Check sheet for the modelled part. Datum: model origin and axes. Units: mm. A direction names the side the tool comes from. Give positions to 0.01 mm unless a question says otherwise; leave off trailing zeros. Loops run counter-clockwise (first coordinate to the right, second up) from the corner with the lowest first, then second, coordinate; pieces in that order, holes last. Notation, with made-up numbers: M 66.25,43.25 L 116.25,43.25 A16 cw 116.25,51.25 Z; hole C -12.75,78.25 d10. An arc over 180 degrees is marked long. Write each question's results on one line, items separated by ' | '. Start each with the question number.
1. Sectioned sample at A-A on y = 38.5. Record the cut outline in (x, z), and give its area (3 significant figures).
2. Tool access check on faces 4 (the flat face through (46, 3, -12.35)), 5 (the flat face through (7, 56, -9)), 6 (the flat face through (-1, 7, -7.5)), 7 (the flat face through (-35, 82, 25)). Record the directions out of +Z, -Z, +X, -X, +Y, -Y that give a thin tool (end or side, any length) a straight path to the whole face; none if there is none.
3. Sectioned sample at B-B on y = 76.5. Record the cut outline in (x, z), and give its area (3 significant figures).
4. Draft check along X on faces 1 (the cylindrical face through (6.3, 56.74, -8.23)), 2 (the flat face through (-30, 87, 30)), 3 (the flat face through (35, 82, -25)). Enter one of: pulls with the +X half, pulls with the -X half, needs draft (parallel to the pull), parting line crosses it, or undercut.
5. Material ranges on line 1 along X through (y, z) = (29, 1); line 2 along X through (y, z) = (60, -33); line 3 along Y through (x, z) = (-31.5, 10), recorded low to high.
6. Go/stop test with flat-tipped pins: pin 1 (3 mm diameter, centred on x = -19.5, z = -3, fed in from -Y); pin 2 (6 mm diameter, centred on x = 12, z = -2, fed in from +Y); pin 3 (3.5 mm diameter, centred on x = 45.5, y = 2.5, fed in from -Z). Record where each tip stops, or that it passes through.
7. Sectioned sample at C-C on y = 13.5. Record the cut outline in (x, z).
8. Sectioned sample at D-D on z = -2. Record the cut outline in (x, y).
```python
from build123d import *

# Parameters (mm, degrees)
SKETCH1_W            = 100
SKETCH1_H            = 100
BOSS_EXTRUDE1_DEPTH  = 25
SKETCH2_W            = 100
SKETCH2_H            = 100
SKETCH2_W_2          = 80
SKETCH2_H_2          = 80
BOSS_EXTRUDE2_DEPTH  = 40
SKETCH3_R            = 5
SKETCH3_W            = 15
SKETCH3_H            = 12
CUT_EXTRUDE1_DEPTH   = 130.325171564
FILLET2_R            = 10
FILLET3_R            = 10
FILLET4_R            = 10
FILLET5_R            = 10
BOSS_EXTRUDE3_DEPTH  = 15
SKETCH6_R            = 35
CUT_EXTRUDE3_DEPTH   = 25
SKETCH7_R            = 40.1
CUT_EXTRUDE4_DEPTH   = 10
BOSS_EXTRUDE4_DEPTH  = 12
SKETCH10_R           = 1.1
SKETCH10_W           = 5
SKETCH10_H           = 13.6
CUT_EXTRUDE5_DEPTH   = 10
FILLET6_R            = 5
SKETCH11_W           = 12
SKETCH11_H           = 0.5
CUT_EXTRUDE6_DEPTH   = 24
SKETCH12_W           = 10
SKETCH12_H           = 15
CUT_EXTRUDE7_DEPTH   = 24
SKETCH15_W           = 10
SKETCH15_H           = 2.75
BOSS_EXTRUDE5_DEPTH  = 5.4
SKETCH18_R           = 2.5
CUT_EXTRUDE8_DEPTH   = 7
BOSS_EXTRUDE6_DEPTH  = 5
FILLET8_R            = 3
FILLET8_OF_MIRROR3_R = 3


with BuildPart() as part:
    # Sketch1 → Boss-Extrude1 (new body)
    with BuildSketch(Plane(origin=(0, 0, 0), x_dir=(1, 0, 0), z_dir=(0, 1, 0))):
        Rectangle(SKETCH1_W, SKETCH1_H)
    extrude(amount=BOSS_EXTRUDE1_DEPTH)

    # Sketch2 → Boss-Extrude2 (add)
    with BuildSketch(Plane(origin=(0, 25, 0), x_dir=(1, 0, 0), z_dir=(0, 1, 0))):
        Rectangle(SKETCH2_W, SKETCH2_H)
        Rectangle(SKETCH2_W_2, SKETCH2_H_2, mode=Mode.SUBTRACT)
    extrude(amount=BOSS_EXTRUDE2_DEPTH)

    # Sketch3 → Cut-Extrude1 (cut, through all)
    with BuildSketch(Plane.ZY.offset(50)):
        with Locations((-25, 12)):
            Circle(SKETCH3_R)
        with Locations((25.313920598, 12)):
            Circle(SKETCH3_R)
        with Locations((0, 6)):
            Rectangle(SKETCH3_W, SKETCH3_H)
    extrude(amount=-CUT_EXTRUDE1_DEPTH, mode=Mode.SUBTRACT)

    # Fillet2
    fillet2_edges = [part.edges().sort_by_distance(p)[0] for p in [
        (50, 32.5, 50),
    ]]
    fillet(fillet2_edges, radius=FILLET2_R)

    # Fillet3
    fillet3_edges = [part.edges().sort_by_distance(p)[0] for p in [
        (50, 32.5, -50),
    ]]
    fillet(fillet3_edges, radius=FILLET3_R)

    # Fillet4
    fillet4_edges = [part.edges().sort_by_distance(p)[0] for p in [
        (-50, 32.5, -50),
    ]]
    fillet(fillet4_edges, radius=FILLET4_R)

    # Fillet5
    fillet5_edges = [part.edges().sort_by_distance(p)[0] for p in [
        (-50, 32.5, 50),
    ]]
    fillet(fillet5_edges, radius=FILLET5_R)

    # Sketch5 → Boss-Extrude3 (add)
    with BuildSketch(Plane(origin=(0, 65, 0), x_dir=(1, 0, 0), z_dir=(0, 1, 0))):
        with BuildLine():
            Line((-50, 40), (-50, -40))
            ThreePointArc((-50, -40), (-47.071067812, -47.071067812), (-40, -50))
            Line((-40, -50), (40, -50))
            ThreePointArc((40, -50), (47.071067812, -47.071067812), (50, -40))
            Line((50, -40), (50, 40))
            ThreePointArc((50, 40), (47.071067812, 47.071067812), (40, 50))
            Line((40, 50), (-40, 50))
            ThreePointArc((-40, 50), (-47.071067812, 47.071067812), (-50, 40))
        make_face()
    extrude(amount=BOSS_EXTRUDE3_DEPTH)

    # Sketch6 → Cut-Extrude3 (cut)
    with BuildSketch(Plane(origin=(0, 80, 0), x_dir=(1, 0, 0), z_dir=(0, 1, 0))):
        with Locations(Location((0.142992369, 0, 0), (0, 0, 270))):
            Circle(SKETCH6_R)
    extrude(amount=-CUT_EXTRUDE3_DEPTH, mode=Mode.SUBTRACT)

    # Sketch7 → Cut-Extrude4 (cut)
    with BuildSketch(Plane(origin=(0, 80, 0), x_dir=(1, 0, 0), z_dir=(0, 1, 0))):
        with Locations(Location((0, 0, 0), (0, 0, 270))):
            Circle(SKETCH7_R)
    extrude(amount=-CUT_EXTRUDE4_DEPTH, mode=Mode.SUBTRACT)

    # Sketch9 → Boss-Extrude4 (add, symmetric)
    with BuildSketch(Plane.XY):
        Polygon((9.8, 56), (9.8, 25), (16.8, 25), (16.8, 58), (4.8, 58), (4.8, 56), align=None)
    boss_extrude4 = extrude(amount=BOSS_EXTRUDE4_DEPTH, both=True)

    # Mirror1: Boss-Extrude4 across plane
    add(boss_extrude4.mirror(Plane.ZY.offset(12.485)))

    # Sketch10 → Cut-Extrude5 (cut)
    with BuildSketch(Plane(origin=(0, 58, 0), x_dir=(1, 0, 0), z_dir=(0, 1, 0))):
        with Locations(Location((8.1, -10.125, 0), (0, 0, 270))):
            Circle(SKETCH10_R)
        with Locations(Location((8.1, 10.125, 0), (0, 0, 270))):
            Circle(SKETCH10_R)
        with Locations((7.3, 0)):
            Rectangle(SKETCH10_W, SKETCH10_H)
    cut_extrude5 = extrude(amount=-CUT_EXTRUDE5_DEPTH, mode=Mode.SUBTRACT)

    # Mirror2: Cut-Extrude5 across plane
    add(cut_extrude5.mirror(Plane.ZY.offset(12.485)), mode=Mode.SUBTRACT)

    # Fillet6
    fillet6_edges = [part.edges().sort_by_distance(p)[0] for p in [
        (-29.77, 57, 6.8),
        (-29.77, 57, -6.8),
        (4.8, 57, 6.8),
        (4.8, 57, -6.8),
    ]]
    fillet(fillet6_edges, radius=FILLET6_R - 0.0001)  # a hair under: the kernel refuses the full size

    # Sketch11 → Cut-Extrude6 (cut)
    with BuildSketch(Plane.XY.offset(12)):
        with Locations((10.8, 57.75)):
            Rectangle(SKETCH11_W, SKETCH11_H)
    extrude(amount=-CUT_EXTRUDE6_DEPTH, mode=Mode.SUBTRACT)

    # Sketch12 → Cut-Extrude7 (cut)
    with BuildSketch(Plane(origin=(0, 25, 0), x_dir=(1, 0, 0), z_dir=(0, 1, 0))):
        with Locations((-12, 0)):
            Rectangle(SKETCH12_W, SKETCH12_H)
    extrude(amount=-CUT_EXTRUDE7_DEPTH, mode=Mode.SUBTRACT)

    # Sketch15 → Boss-Extrude5 (add)
    with BuildSketch(Plane(origin=(0, 25, 0), x_dir=(1, 0, 0), z_dir=(0, 1, 0))):
        with Locations((-12.485, -10.625)):
            Rectangle(SKETCH15_W, SKETCH15_H)
    extrude(amount=BOSS_EXTRUDE5_DEPTH)

    # Sketch18 → Cut-Extrude8 (cut)
    # profile 1 of 2: a face of its own
    with BuildSketch(Plane.XZ):
        with BuildLine():
            Line((-50, -12.35), (-50, -14.65))
            Line((-50, -14.65), (-41.831122551, -14.65))
            ThreePointArc((-41.831122551, -14.65), (-34, -13.5), (-41.831122551, -12.35))
            Line((-41.831122551, -12.35), (-50, -12.35))
        make_face()
        with Locations(Location((-38, -13.5, 0), (0, 0, 270))):
            Circle(SKETCH18_R, mode=Mode.SUBTRACT)
    # profile 2 of 2: a face of its own
    with BuildSketch(Plane.XZ):
        with BuildLine():
            Line((41.845776905, -14.65), (50, -14.65))
            Line((50, -14.65), (50, -12.35))
            Line((50, -12.35), (41.845776905, -12.35))
            ThreePointArc((41.845776905, -12.35), (33.985962133, -13.5), (41.845776905, -14.65))
        make_face()
        with Locations(Location((38, -13.5, 0), (0, 0, 90))):
            Circle(SKETCH18_R, mode=Mode.SUBTRACT)
    extrude(amount=-CUT_EXTRUDE8_DEPTH, mode=Mode.SUBTRACT)

    # Sketch20 → Boss-Extrude6 (add)
    with BuildSketch(Plane(origin=(-28.354981926, 0, 28.354981926), x_dir=(0.7071067811865476, 0, 0.7071067811865475), z_dir=(-0.7071067811865475, 0, 0.7071067811865476))):
        Polygon((-4.498932188, 80), (-4.498932188, 84), (4.501067812, 84), (4.501067812, 80), (7.071067812, 80), (7.071067812, 87), (-7.071067812, 87), (-7.071067812, 80), align=None)
    boss_extrude6 = extrude(amount=BOSS_EXTRUDE6_DEPTH)

    # Fillet8
    fillet8_edges = [part.edges().sort_by_distance(p)[0] for p in [
        (-35.122748879, 87, 25.122748879),
        (-25.122748879, 87, 35.122748879),
    ]]
    fillet(fillet8_edges, radius=FILLET8_R)

    # Mirror3: Boss-Extrude6 across plane
    add(boss_extrude6.mirror(Plane(origin=(0, 0, 0), x_dir=(0.7071067811865476, 0, 0.7071067811865475), z_dir=(-0.7071067811865475, 0, 0.7071067811865476))))

    # Fillet8 of Mirror3
    fillet8_of_mirror3_edges = [part.edges().sort_by_distance(p)[0] for p in [
        (25.122748879, 87, -35.122748879),
        (35.122748879, 87, -25.122748879),
    ]]
    fillet(fillet8_of_mirror3_edges, radius=FILLET8_OF_MIRROR3_R)


solid = part.part
```
Output values:
1) outline: M -50,-40 A10 ccw -40,-50 L 40,-50 A10 ccw 50,-40 L 50,40 A10 ccw 40,50 L -40,50 A10 ccw -50,40 Z; M 9.8,-12 L 16.8,-12 L 16.8,12 L 9.8,12 Z; hole M -40,-40 L 40,-40 L 40,40 L -40,40 L -40,12 L -34.77,12 L -34.77,-12 L -40,-12 Z | area: 3,810 mm2
2) face 4: +X, -Y | face 5: none | face 6: -Y | face 7: -Z, -X, +Y
3) outline: M -50,-40 A10 ccw -40,-50 L 40,-50 A10 ccw 50,-40 L 50,40 A10 ccw 40,50 L -40,50 A10 ccw -50,40 Z; hole C 0,0 d80.2 | area: 4,860 mm2
4) face 1: undercut | face 2: needs draft | face 3: pulls with the +X half
5) line 1: -50 to -34.77, 9.8 to 16.8, 40 to 50 | line 2: -50 to -40, 40 to 50 | line 3: 0 to 25, 56 to 58
6) pin 1: y = 12 | pin 2: y = 57.5 | pin 3: z = -49.27
7) outline: M -50,-40 A10 ccw -40,-50 L 40,-50 A10 ccw 50,-40 L 50,-29.77 L -50,-29.77 Z; M -50,-20.23 L 50,-20.23 L 50,20.54 L -50,20.54 Z; M -50,30.08 L 50,30.08 L 50,40 A10 ccw 40,50 L -40,50 A10 ccw -50,40 Z; hole M -17,-7.5 L -7,-7.5 L -7,7.5 L -17,7.5 Z
8) outline: M -50,12 L -17,12 L -17,25 L -34.77,25 L -34.77,58 L -40,58 L -40,65 L -34.8,65 L -34.8,70 L -40.05,70 L -40.05,80 L -50,80 Z; M -7,12 L 50,12 L 50,80 L 40.05,80 L 40.05,70 L 35.09,70 L 35.09,65 L 40,65 L 40,25 L 16.8,25 L 16.8,57.5 L 9.8,57.5 L 9.8,25 L -7,25 Z
